Geometry: final body of the model. Coordinates: model frame, mm. Coordinates: 2 decimals unless noted, no trailing zeros. Order: outer loops, then holes, each group sorted by start corner. A loop starts at its lowest first (then second) coordinate and runs counter-clockwise, first axis right, second up. Notation, with made-up numbers: M -8,57 L 14,57 A8 cw 14,61 Z; hole C -25.75,-28.5 d9. An arc over 180 degrees is marked long. Write item = value, one per line.
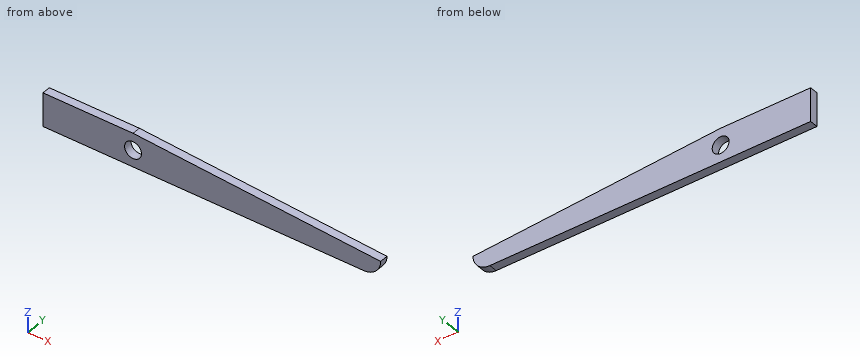
from build123d import *

# Parameters (mm, degrees)
F0_R     = 1.5
F1_DEPTH = 1.5


with BuildPart() as f1:
    # F0 (on Front) → F1 (new body)
    with BuildSketch(Plane.XZ):
        with BuildLine():
            Line((0, 3), (-16, 3))
            Line((-16, 3), (-16, -3))
            Line((-16, -3), (41, -3))
            ThreePointArc((41, -3), (43.12132, -2.12132), (44, 0))
            Line((44, 0), (0, 3))
        make_face()
        Circle(F0_R, mode=Mode.SUBTRACT)
    extrude(amount=F1_DEPTH)


solid = f1.part
1) Section C-C, the plane x = 6. Return loops of the section in (y, z), and give its area (3 significant figures).
Numbers:
outline = M -1.5,-3 L 0,-3 L 0,2.59 L -1.5,2.59 Z
area = 8.39 mm²
2) Section B-B, the plane y = -0.45. Return loops of the section in (x, z), and give its area (3 significant figures).
Numbers:
outline = M -16,-3 L 41,-3 A3 ccw 44,0 L 0,3 L -16,3 Z; hole C 0,0 d3
area = 285 mm²
3) Section A-A, the plane z = 1. Return loops of the section in (x, y), and give its area (3 significant figures).
Numbers:
outline = M -16,-1.5 L -1.12,-1.5 L -1.12,0 L -16,0 Z; M 1.12,-1.5 L 29.33,-1.5 L 29.33,0 L 1.12,0 Z
area = 64.6 mm²
4) Line query: L1, parallel to Z at x = 0, y = -0.85; L2, parallel to X at y = -1.2, z = -1; L3, parallel to X at y = -0.35, z = -1.25. Output: solid intervals per line, ascending.
Numbers:
L1 = -3 to -1.5, 1.5 to 3
L2 = -16 to -1.12, 1.12 to 43.83
L3 = -16 to -0.83, 0.83 to 43.73
5) Section D-D, the plane z = -2.25. Return loops of the section in (x, y).
Numbers:
outline = M -16,-1.5 L 42.98,-1.5 L 42.98,0 L -16,0 Z
